Geometry: final body of the model. Coordinates: model frame, mm. A direction names the side the tool comes from. Give positions to 0.01 mm unless a question says otherwise; leave off trailing zeros. Write each loop counter-clockwise with the first axis right and the second up, starting at its lowest first coordinate (ties: lowest second). Pieces come first, ordered by that corner, then holes.
Q1. Section B-B (x = -253.5). Return the cut outline in (y, z), plus the area to 3 significant figures.
Q2. Mould query, pull axis Z, two halves, no side actions, for faces 3 (the flat face through (-4, 114, 100)), 4 (the cylindrical face through (-295.49, 114.2, -95.72)), 5 (the flat face through (285, 122, -1)). Classes: +Z half, -Z half, draft (parallel to the pull), parting line (faces both ways), or undercut.
Q3. Reachability of faces 1 (the flat face through (-285, 122, 1)), 2 (the flat face through (-1, 225, 88)) from +Z, -Z, +X, -X, +Y, -Y: full face, straight path, thin tool, end or side. Return the list, or none.
Q4. Section A-A (y = 198). Return the cut outline in (x, z).
Q5. Line query: line 1 (X direction, y = 73, z = 9.5); line 2 (Z direction, x = -136, y = 183.5); line 3 (Y direction, x = -170, z = -29). Output: solid intervals per line, ascending.
Q6. Section C-C (z = 16.5). Return the cut outline in (x, y).
Autodesk Inventor part; units mm, degrees
ref_plane "YZ Plane" through (0, 0, 0) normal (1, 0, 0) x (0, 1, 0)
ref_plane "XZ Plane" through (0, 0, 0) normal (0, 1, 0) x (-1, 0, 0)
ref_plane "XY Plane" through (0, 0, 0) normal (0, 0, 1) x (1, 0, 0)
sketch "Skizze1" plane through (0, 0, 0) normal (0, 0, 1) x (1, 0, 0)
  line L0 (-300, 0.252) -> (300, 0.252)
  line L1 (300, 0.252) -> (300, 250.252)
  line L2 (300, 250.252) -> (-300, 250.252)
  line L3 (-300, 250.252) -> (-300, 0.252)
  point P0 (0, 0)
  dimension "d0" = 600
  dimension "d1" = 250
extrude "Extrusion1" add sketch "Skizze1" along normal mid plane 200
sketch "Skizze2" plane through (-300, 250.252, 100) normal (0, 1, 0) x (1, 0, 0)
  line L0 (600, 0) -> (0, 0)
  line L1 (600, 200) -> (600, 0)
  line L2 (15, 0) -> (585, 0)
  line L3 (600, 15) -> (600, 185)
  line L4 (585, 200) -> (15, 200)
  line L5 (0, 185) -> (0, 15)
  arc A0 (0, 15) -> (15, 0) centre (15, 15) ccw
  arc A1 (15, 200) -> (0, 185) centre (15, 185) ccw
  arc A2 (600, 185) -> (585, 200) centre (585, 185) ccw
  arc A3 (585, 0) -> (600, 15) centre (585, 15) ccw
  line L6 (0, 200) -> (0, 0)
  line L7 (0, 200) -> (600, 200)
  line L8 (0, 0) -> (600, 0)
  line L9 (600, 0) -> (600, 200)
  line L10 (600, 200) -> (0, 200)
  line L11 (0, 200) -> (0, 0)
  point P0 (300, 100)
  point P1 (585, 0)
  dimension "d4" = 15
extrude "Extrusion2" cut sketch "Skizze2" against normal through all contours L0 A3 L1 | L0 L6 A0 | A2 L7 L1 | L6 L7 A1
sketch "Skizze3" plane through (-285, 250.252, 100) normal (0, 1, 0) x (1, 0, 0)
  arc A0 (0, 200) -> (-15, 185) centre (0, 185) ccw
  arc A1 (570, 0) -> (585, 15) centre (570, 15) ccw
  line L0 (0, 185) -> (570, 185)
  line L1 (570, 185) -> (570, 15)
  line L2 (570, 15) -> (0, 15)
  line L3 (0, 15) -> (0, 185)
  point P0 (285, 100)
extrude "Extrusion3" cut sketch "Skizze3" against normal blind 235
sketch "Skizze4" plane through (0, 0, 0) normal (1, 0, 0) x (0, 1, 0)
  line L0 (225, 85) -> (225, -110.1417)
  line L1 (250.252, -85) -> (15.252, -85)
  line L2 (225, 85) -> (225, 112.4289)
  line L3 (225, 112.4289) -> (265.8438, 112.4289)
  line L4 (265.8438, 112.4289) -> (265.8438, -110.1417)
  line L5 (265.8438, -110.1417) -> (225, -110.1417)
  point P0 (0, 0)
extrude "Extrusion4" cut sketch "Skizze4" along normal through all both and the other way through all
properties part number "beetkasten"
Computed:
1. outline: (0.25, -100) - (225, -100) - (225, -85) - (15.25, -85) - (15.25, 85) - (225, 85) - (225, 100) - (0.25, 100) - close
1. area: 9,290 mm2
2. face 3: +Z half
2. face 4: -Z half
2. face 5: undercut
3. face 1: +Y
3. face 2: +Z, -Z, +X, -X, +Y
4. outline: (-300, -85) arc R15 ccw to (-285, -100) - (285, -100) arc R15 ccw to (300, -85) - (300, 85) arc R15 ccw to (285, 100) - (-285, 100) arc R15 ccw to (-300, 85) - close; hole (-285, -85) - (285, -85) - (285, 85) - (-285, 85) - close
5. line 1: x = -300 to -285, 285 to 300
5. line 2: z = -100 to -85, 85 to 100
5. line 3: y = 0.25 to 15.25
6. outline: (-300, 0.25) - (300, 0.25) - (300, 225) - (285, 225) - (285, 15.25) - (-285, 15.25) - (-285, 225) - (-300, 225) - close
